Design review of the part built by this model. Coordinates are the model's own, in mm. Face numbers are marked on the shaded views. A direction names the side the tool comes from. Give positions to 0.01 mm unless a question says otherwise; leave off trailing zeros. Loops run counter-clockwise (first coordinate to the right, second up) from the corner with the lowest first, then second, coordinate; pieces in that order, holes last.
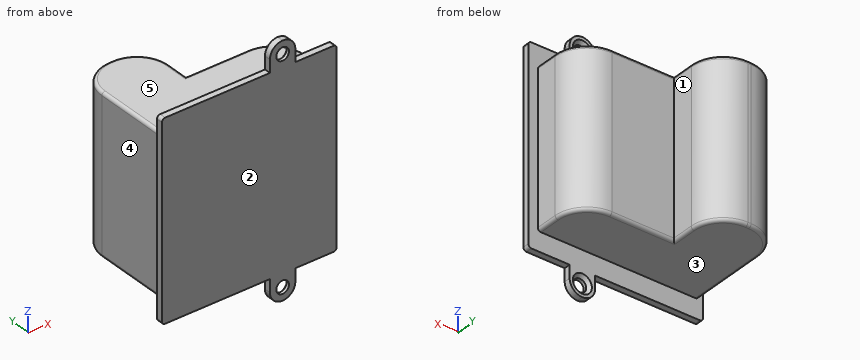
from build123d import *

# Parameters (mm, degrees)
BOSS_EXTRUDE1_DEPTH = 49
FILLET1_R           = 10
FILLET2_R           = 1
SKETCH2_W           = 55
SKETCH2_H           = 6
SKETCH2_W_2         = 8
SKETCH2_H_2         = 8
SKETCH2_R           = 2
BOSS_EXTRUDE2_DEPTH = 2
FILLET3_R           = 4
FILLET4_R           = 1
CHAMFER1_SIZE       = 1


with BuildPart() as part:
    # Sketch1 → Boss-Extrude1 (new body)
    with BuildSketch(Plane.XY):
        Polygon((0, 0), (55, 0), (55, 2), (52.011494253, 2), (52.011494253, 19), (22.471264368, 19), (22.471264368, 36), (1.436781609, 36), (1.436781609, 2), (0, 2), align=None)
    extrude(amount=BOSS_EXTRUDE1_DEPTH)

    # Fillet1
    fillet1_edges = [part.edges().sort_by_distance(p)[0] for p in [
        (1.436781609, 36, 24.5),
        (22.471264368, 36, 24.5),
        (52.011494253, 19, 24.5),
    ]]
    fillet(fillet1_edges, radius=FILLET1_R)

    # Fillet2
    fillet2_edges = [part.edges().sort_by_distance(p)[0] for p in [
        (22.471264368, 22.5, 0),
        (52.011494253, 5.5, 0),
        (52.011494253, 5.5, 49),
        (22.471264368, 22.5, 49),
        (32.24137931, 19, 0),
        (32.24137931, 19, 49),
        (1.436781609, 14, 0),
        (11.954022989, 36, 0),
        (19.54233218, 33.071067812, 0),
        (4.365713797, 33.071067812, 0),
        (49.082562065, 16.071067812, 0),
        (11.954022989, 36, 49),
        (1.436781609, 14, 49),
        (19.54233218, 33.071067812, 49),
        (4.365713797, 33.071067812, 49),
        (49.082562065, 16.071067812, 49),
    ]]
    fillet(fillet2_edges, radius=FILLET2_R)

    # Sketch2 → Boss-Extrude2 (add)
    # profile 1 of 2: a face of its own
    with BuildSketch(Plane.XZ):
        with Locations((27.5, 52)):
            Rectangle(SKETCH2_W, SKETCH2_H)
    # profile 2 of 2: a face of its own
    with BuildSketch(Plane.XZ):
        with Locations((38, 59)):
            Rectangle(SKETCH2_W_2, SKETCH2_H_2)
        with Locations(Location((38, 59, 0), (0, 0, 270))):
            Circle(SKETCH2_R, mode=Mode.SUBTRACT)
    extrude(amount=-BOSS_EXTRUDE2_DEPTH)

    # Fillet3
    fillet3_edges = [part.edges().sort_by_distance(p)[0] for p in [
        (34, 1, 63),
        (42, 1, 63),
    ]]
    fillet(fillet3_edges, radius=FILLET3_R - 0.0001)  # a hair under: the kernel refuses the full size

    # Fillet4
    fillet4_edges = [part.edges().sort_by_distance(p)[0] for p in [
        (0, 1, 55),
        (55, 1, 55),
    ]]
    fillet(fillet4_edges, radius=FILLET4_R)

    # Mirror7: part across plane


with BuildPart() as part_1:
    add(part.part)
    add(part.part.mirror(Plane.XY.offset(24.5)))

    # Chamfer1
    chamfer1_edges = [part_1.edges().sort_by_distance(p)[0] for p in [
        (38, 2, 61),
        (38, 2, -12),
    ]]
    chamfer(chamfer1_edges, length=CHAMFER1_SIZE)


solid = part_1.part
Q1. Wall thickness on line 1 (X direction, y = 0.65, z = 59); line 2 (Y direction, x = 6.5, z = 53); line 3 (Z direction, x = 43, y = 11): over which ranges is each line inside the solid? List them lowest first.
Results:
line 1: x = 34 to 36, 40 to 42
line 2: y = 0 to 2
line 3: z = 0 to 49
Q2. Tool access review of the marked faces 1, 2, 3, 4 and 5: name each direction out of +Z, -Z, +X, -X, +Y, -Y from which nothing blocks a thin tool from reaching the whole face with its end or side.
Results:
face 1: +Z, -Z, +X, +Y
face 2: +Z, -Z, +X, -X, -Y
face 3: -Z, +X, -X, +Y
face 4: +Z, -Z, -X, +Y
face 5: +Z, +X, -X, +Y
Q3. Insertion check: pin 1 (10 mm diameter, centred on x = 16.5, y = 11, fed in from -Z); pin 2 (3 mm diameter, centred on x = 22.5, z = 35.5, fed in from +Y); pin 3 (10 mm diameter, centred on x = 47.5, y = 10.5, fed in from +Z); pin 4 (2.5 mm diameter, centred on x = 38, z = 59, fed in from +Y). Each pin has a flat end and moves straight along its axis. Give the tip position at first contact, or say it passes through.
Results:
pin 1: stops at z = 0
pin 2: stops at y = 31.22
pin 3: stops at z = 49
pin 4: passes through
Q4. Take a section at B-B (x = 26). Give the boundary of the cut face in (y, z), plus the area to 3 significant figures.
Results:
outline: (0, -6) - (2, -6) - (2, 0) - (18, 0) arc R1 ccw to (19, 1) - (19, 48) arc R1 ccw to (18, 49) - (2, 49) - (2, 55) - (0, 55) - close
area: 955 mm2
Q5. Take a section at A-A (z = 12). Give the boundary of the cut face in (x, y).
Results:
outline: (0, 0) - (55, 0) - (55, 2) - (52.01, 2) - (52.01, 9) arc R10 ccw to (42.01, 19) - (22.47, 19) - (22.47, 26) arc R10 ccw to (12.47, 36) - (11.44, 36) arc R10 ccw to (1.44, 26) - (1.44, 2) - (0, 2) - close
